The figure shows three views and two pictorial views of one solid part (mm, origin at its lowest corner). Answer the questions. Give positions to 0.01 mm unless a question says otherwise; leave off trailing zeros. Write each loop counter-clockwise with the first axis right and the second up, starting at its lowest first coordinate (ties: lowest second). Pieces come first, ordered by that corner, then holes. Notation, with made-up numbers: M 9.25,72 L 30.25,72 A28 cw 30.25,90 Z; hole C 40.25,81.25 d8. An arc over 180 degrees is marked long. Answer as CSV lines item,"result". Start each with the question number.
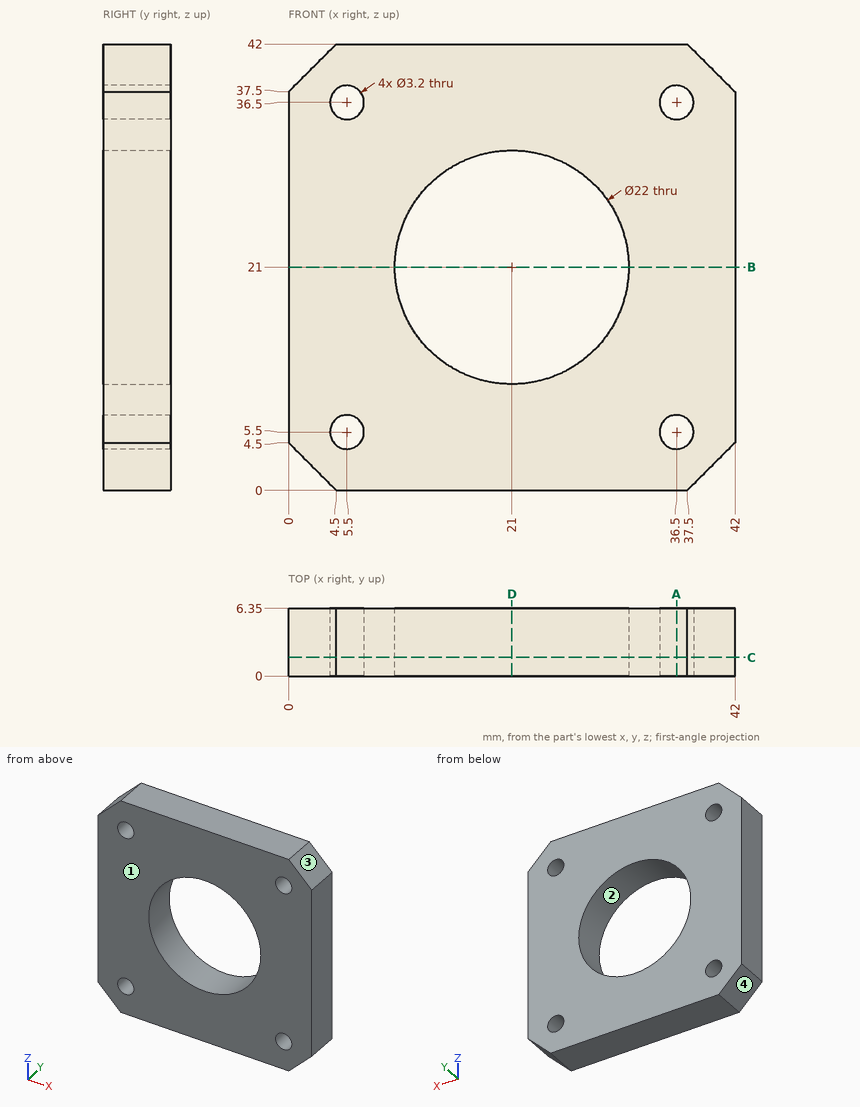
1. Find section A-A on x = 36.5. Determine the outline of the cut face in (y, z), then the cut area to 3 significant figures.
2. Given pin 1 (4 mm diameter, centred on x = 36.5, z = 36.5, fed in from +Y); pin 2 (1.9 mm diameter, centred on x = 5.5, z = 5.5, fed in from +Y), each flat-ended and moving along its own axis, determine where each tip first touches the part or whether it passes through.
3. Find section C-C on y = 1.75. Determine the outline of the cut face in (x, z), then the cut area to 3 significant figures.
4. Find section B-B on z = 21. Determine the outline of the cut face in (x, y), then the cut area to 3 significant figures.
5. Find section D-D on x = 21. Determine the outline of the cut face in (y, z), then the cut area to 3 significant figures.
6. Determine the mould class of the marked faces 1, 2, 3 and 4 for opening direction X: +X half, -X half, draft (parallel to the pull), parting line (faces both ways), or undercut.
7. Find the intervals of material crossed by line 1 (Z direction, x = 36.5, y = 2.75); line 2 (X direction, y = 5, z = 21), in increasing order. Write a range as [from, to].
Computed:
1,outline,"M 0,0 L 6.35,0 L 6.35,3.9 L 0,3.9 Z; M 0,7.1 L 6.35,7.1 L 6.35,34.9 L 0,34.9 Z; M 0,38.1 L 6.35,38.1 L 6.35,42 L 0,42 Z"
1,area,"226 mm^2"
2,pin 1,"stops at y = 6.35"
2,pin 2,"passes through"
3,outline,"M 0,4.5 L 4.5,0 L 37.5,0 L 42,4.5 L 42,37.5 L 37.5,42 L 4.5,42 L 0,37.5 Z; hole C 5.5,5.5 d3.2; hole C 5.5,36.5 d3.2; hole C 21,21 d22; hole C 36.5,5.5 d3.2; hole C 36.5,36.5 d3.2"
3,area,"1,310 mm^2"
4,outline,"M 0,0 L 10,0 L 10,6.35 L 0,6.35 Z; M 32,0 L 42,0 L 42,6.35 L 32,6.35 Z"
4,area,"127 mm^2"
5,outline,"M 0,0 L 6.35,0 L 6.35,10 L 0,10 Z; M 0,32 L 6.35,32 L 6.35,42 L 0,42 Z"
5,area,"127 mm^2"
6,face 1,"draft"
6,face 2,"undercut"
6,face 3,"+X half"
6,face 4,"-X half"
7,line 1,"z = [0, 3.9], [7.1, 34.9], [38.1, 42]"
7,line 2,"x = [0, 10], [32, 42]"
